Work out the finished part from the listing and answer in its coordinate system (mm). Give positions to 0.01 mm unless a question says otherwise; leave off trailing zeros. Loops run counter-clockwise (first coordinate to the right, second up) from the corner with the lowest first, then second, coordinate; pieces in that order, holes last. Notation, with made-up numbers: (-39.75, -34) - (-32.75, -34) arc R8 ccw to (-32.75, -21) - close; hole circle Ø8 at (42, 25). An arc over 180 degrees is marked (long way). One line per item, written item: value.
Autodesk Inventor part; units mm, degrees
ref_plane "YZ Plane" through (0, 0, 0) normal (1, 0, 0) x (0, 1, 0)
ref_plane "XZ Plane" through (0, 0, 0) normal (0, 1, 0) x (-1, 0, 0)
ref_plane "XY Plane" through (0, 0, 0) normal (0, 0, 1) x (1, 0, 0)
sketch "Sketch1" plane through (0, 0, 0) normal (0, 1, 0) x (-1, 0, 0)
  circle A0 centre (0, 0) radius 3
  dimension "d0" = 6
extrude "Extrusion1" add sketch "Sketch1" along normal blind 120
sketch "Sketch2" plane through (0, 120, 0) normal (0, 1, 0) x (1, 0, 0)
  circle A0 centre (0, 0) radius 3
  circle A1 centre (0, 0) radius 3
  line L0 (-2.5981, 1.5) -> (2.5981, 1.5)
  line L1 (2.5981, -1.5) -> (-2.5981, -1.5)
  line L2 (0, -1.5) -> (0, 1.5)
  dimension "d3" = 3
extrude "Extrusion2" add sketch "Sketch2" along normal blind 7 contours A0 L1 L2 L0 | L0 L2 L1 A0
sketch "Sketch3" plane through (-2.5981, 120, 1.5) normal (0, 0, 1) x (1, 0, 0)
  line L0 (5.5981, -120) -> (5.5981, 7)
  line L1 (-0.4019, -120) -> (-0.4019, 7)
  line L2 (-0.4019, 4) -> (5.5981, 4)
  circle A0 centre (2.5981, 4) radius 2
  line L3 (0, 7) -> (5.1962, 7)
  circle A1 centre (2.5981, 4) radius 3
  line L4 (0, 7) -> (-0.4019, 7)
  line L5 (-0.4019, 7) -> (5.5981, 7)
  point P0 (2.5981, -120)
  point P1 (2.5981, 7)
  point P2 (5.5981, 4)
  dimension "d6" = 4
extrude "Extrusion3" cut sketch "Sketch3" against normal blind 7 contours A1 L3 L5 L0 | A0 L2 | L2 A0 | L1 L4 L3 A1
properties part number "Shaft"
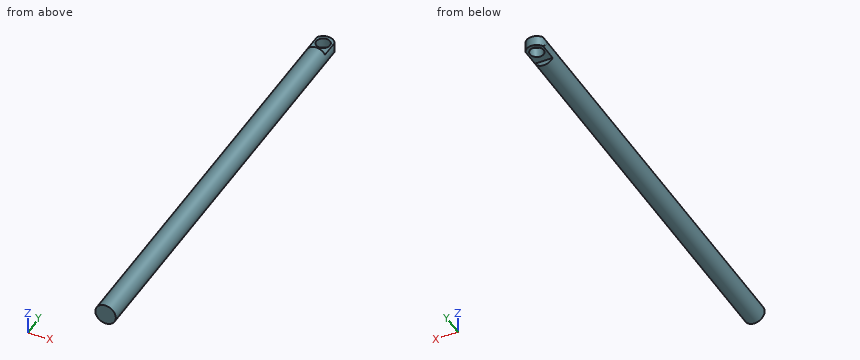
1. Section B-B (y = 114) is taken. Write down the section's boundary in (x, z), and give its area (3 significant figures).
Output:
outline: circle Ø6 at (0, 0)
area: 28.3 mm²
2. Find the intervals of material crossed by line 1 along Z through (x, y) = (-2.25, 41); line 2 along X through (y, z) = (116, -0.35); line 3 along Y through (x, z) = (0.9, -1.85), in increasing order.
Output:
line 1: z = -1.98 to 1.98
line 2: x = -2.98 to 2.98
line 3: y = 0 to 120
3. Section A-A (x = 0) is taken. Write down the section's boundary in (y, z).
Output:
outline: (0, -3) - (120, -3) - (120, -1.5) - (122, -1.5) - (122, 1.5) - (120, 1.5) - (120, 3) - (0, 3) - close; (126, -1.5) - (127, -1.5) - (127, 1.5) - (126, 1.5) - close
4. Flat-ended cylindrical pins translate along their axes: pin 1 Ø3 at (x, z) = (-0.5, -1) entering from -Y; pin 2 Ø0.5 at (x, z) = (1, 2.5) entering from +Y; pin 3 Ø1.6 at (x, y) = (-1, 125) entering from +Z; pin 4 Ø1.6 at (x, y) = (-1.5, 124) entering from -Z. Find the tip coordinate at first contact, or state that the pin passes through.
Output:
pin 1: stops at y = 0
pin 2: stops at y = 120
pin 3: stops at z = 1.5
pin 4: stops at z = -1.5
